from build123d import *

# Parameters (mm, degrees)
RESSALTO_EXTRUS_O1_DEPTH = 50
CASCA1_T                 = -3
ESBO_O4_R                = 1.6
ESBO_O4_R_2              = 5
ESBO_O4_R_3              = 3
ESBO_O4_R_4              = 2.5
ESBO_O4_W                = 79
ESBO_O4_H                = 51.6
CORTE_EXTRUS_O1_DEPTH    = 3


with BuildPart() as part:
    # Esboço2 → Ressalto-extrusão1 (new, symmetric)
    with BuildSketch(Plane(origin=(0, 0, 0), x_dir=(0, 0, -1), z_dir=(1, 0, 0))):
        Polygon((0, 0), (70.09159675, 0), (70.09159675, 10), (10, 77), (0, 77), align=None)
    extrude(amount=RESSALTO_EXTRUS_O1_DEPTH, both=True)

    # Casca1
    casca1_openings = [part.faces().sort_by_distance(p)[0] for p in [
        (0, 0, -35.045798375),
        (0, 38.5, 0),
    ]]
    offset(amount=CASCA1_T, openings=casca1_openings, kind=Kind.INTERSECTION)

    # Esboço4 → Corte-extrusão1 (cut)
    with BuildSketch(Plane(origin=(0, 39.297329608, -43.815129338), x_dir=(1, 0, 0), z_dir=(0, 0.6676844083366051, -0.7444444444444445))):
        with Locations(Location((-44, 19.854621861, 0), (0, 0, 270))):
            Circle(ESBO_O4_R)
        with Locations(Location((-44, -45.145378139, 0), (0, 0, 270))):
            Circle(ESBO_O4_R)
        with Locations(Location((44, -45.145378139, 0), (0, 0, 270))):
            Circle(ESBO_O4_R)
        with Locations(Location((44, 19.854621861, 0), (0, 0, 270))):
            Circle(ESBO_O4_R)
        with Locations(Location((-37.5, 30.654621861, 0), (0, 0, 270))):
            Circle(ESBO_O4_R_2)
        with Locations(Location((36.75, 28.054621861, 0), (0, 0, 270))):
            Circle(ESBO_O4_R_3)
        with Locations(Location((-3.8, 31.054621861, 0), (0, 0, 270))):
            Circle(ESBO_O4_R_4)
        with Locations((0, -12.845378139)):
            Rectangle(ESBO_O4_W, ESBO_O4_H)
    extrude(amount=-CORTE_EXTRUS_O1_DEPTH, mode=Mode.SUBTRACT)


solid = part.part
Work out the finished part from the listing and answer in its coordinate system (mm). A direction names the side the tool comes from. Give positions to 0.01 mm unless a question says otherwise; leave off trailing zeros. Order: outer loops, then holes, each group sorted by start corner. A loop starts at its lowest first (then second) coordinate and runs counter-clockwise, first axis right, second up. Notation, with made-up numbers: (-18.75, 28.5) - (2.25, 28.5) arc R23 cw to (2.25, 44.5) - close; hole circle Ø1 at (-13, -23.75). An arc over 180 degrees is marked (long way). Answer as CSV lines item,"result". Start each with the question number.
Q1. Find the intervals of material crossed by L1, parallel to X at y = 63, z = -19.5; L2, parallel to X at y = 47.5, z = -8; L3, parallel to Y at x = -27.5, z = -7, in increasing order. Write a range as [from, to].
Q2. The part is cut by section D-D (y = 7). Write down the section's boundary in (x, z), then the cut area to 3 significant figures.
Q3. The part is cut by section A-A (x = -21). Write down the section's boundary in (y, z), then the cut area to 3 significant figures.
Q4. Given pin 1 Ø1.5 at (x, z) = (-8, -16.5) entering from -Y; pin 2 Ø6 at (x, y) = (6.5, 28.5) entering from +Z; pin 3 Ø4 at (x, z) = (4, -57) entering from +Y, each flat-ended and moving along its own axis, determine where each tip first touches the part or whether it passes through.
Q5. For faces 1 (the face through (-0.6, 28.7, -51.4)), 2 (the face through (1, 77, -5)), 3 (the face through (-0.55, 67.08, -16.91)), 4 (the face through (0.66, 26.49, -51.27)), determine the directions among +Z, -Z, +X, -X, +Y, -Y from which every point of the face is accessible in a straight line to the end or side of a thin tool.
Q6. The part is cut by section C-C (z = -5.5). Write down the section's boundary in (x, y).
Q7. The mould has two halves that part along Z. Classify faces 5 (the face through (0, 76, 0)), 6 (the face through (39.5, 48, -34)), 7 (the face through (-43.93, 22.34, -57.04)): +Z half, -Z half, draft (parallel to the pull), parting line (faces both ways), or undercut.
Q8. The part is cut by section B-B (z = -25.5). Write down the section's boundary in (x, y).
Check result:
1,L1,"x = [-50, -39.5], [39.5, 50]"
1,L2,"x = [-50, -47], [47, 50]"
1,L3,"y = [74, 77]"
2,outline,"(-50, -70.09) - (50, -70.09) - (50, 0) - (47, 0) - (47, -67.09) - (-47, -67.09) - (-47, 0) - (-50, 0) - close"
2,area,"703 mm²"
3,outline,"(0, -70.09) - (10, -70.09) - (29.65, -52.46) - (27.65, -50.23) - (8.85, -67.09) - (0, -67.09) - close; (66.06, -15.78) - (68.07, -18.01) - (77, -10) - (77, 0) - (74, 0) - (74, -8.66) - close"
3,area,"168 mm²"
4,pin 1,"stops at y = 66.06"
4,pin 2,"stops at z = -50.23"
4,pin 3,"stops at y = 26.83"
5,face 1,"+Z, +Y"
5,face 2,"+Z, -Z, +X, -X, +Y"
5,face 3,"-Z, -Y"
5,face 4,"+Z, -Y"
6,outline,"(-50, 0) - (-47, 0) - (-47, 74) - (47, 74) - (47, 0) - (50, 0) - (50, 77) - (-50, 77) - close"
7,face 5,"+Z half"
7,face 6,"draft"
7,face 7,"undercut"
8,outline,"(-50, 0) - (-47, 0) - (-47, 55.22) - (-39.5, 55.22) - (-39.5, 59.72) - (-50, 59.72) - close; (39.5, 55.22) - (47, 55.22) - (47, 0) - (50, 0) - (50, 59.72) - (39.5, 59.72) - close"
